Can you work these out from the model? Positions are in its coordinate system, mm. A direction names the side the tool comes from. Round coordinates to 2 decimals unless told otherwise and drop trailing zeros. Loops run counter-clockwise (first coordinate to the right, second up) from the corner with the lowest first, then second, coordinate; pieces in that order, holes last.
(1) If I drill on line 1 along X through (y, z) = (-6.5, -4.25); line 2 along Z through (x, y) = (6.5, -4.5); line 3 along X through (y, z) = (-7.5, -4), over which ranges is the centre line in solid material (lowest first)?
(2) I want a section at D-D on y = -0.5. Write out the boundary of the cut face in (x, z).
(3) Will this pin go through, and if not, where does the flat tip stop? pin 1 Ø1.5 at (x, y) = (-5, -6.5) entering from -Z.
(4) I want a section at A-A on z = -6. Write out the boundary of the cut face in (x, y), plus the area to 3 significant figures.
(5) I want a section at B-B on x = -1. Write out the boundary of the cut face in (y, z), plus the area to 3 significant figures.
(6) I want a section at C-C on y = -3.75. Write out the boundary of the cut face in (x, z).
(7) Thinking about a two-plate mould opening in X: for faces 1 (the face through (-12.458, -7.699, -7.715)), 2 (the face through (0.105, -7.715, 0.301)), 3 (the face through (16.199, -0.285, 0.098)), which applies, released by +X, released by -X, zero draft, split by the parting line, or undercut?
(8) Which directions (+Z, -Z, +X, -X, +Y, -Y) give clear straight access to the entire face, cutting with the end or side of a thin tool? Please do faces 4 (the face through (0, -4, 0)), 5 (the face through (0, 0, 2)), 6 (the face through (8.801, -0.285, -3.958)).
from build123d import *

# Parameters (mm, degrees)
F0_W     = 33
F0_H     = 16
F1_DEPTH = 8
F2_W     = 17
F2_H     = 8
F3_DEPTH = 25
F4_R     = 1


with BuildPart() as f1:
    # F0 (on Front) → F1 (new body)
    with BuildSketch(Plane.XZ):
        Rectangle(F0_W, F0_H)
    extrude(amount=F1_DEPTH)

    # F2 (on face) → F3 (cut)
    with BuildSketch(Plane.XZ.offset(8)):
        with Locations((0, -4)):
            Rectangle(F2_W, F2_H)
    extrude(amount=-F3_DEPTH, mode=Mode.SUBTRACT)

    # F4
    f4_edges = [f1.edges().sort_by_distance(p)[0] for p in [
        (16.5, -8, 0),
        (12.5, -8, -8),
        (8.5, -8, -4),
        (0, -8, 0),
        (-8.5, -8, -4),
        (-12.5, -8, -8),
        (-16.5, -8, 0),
        (0, -8, 8),
        (-8.5, 0, -4),
        (16.5, 0, 0),
        (12.5, 0, -8),
        (8.5, 0, -4),
        (0, 0, 0),
        (-12.5, 0, -8),
        (-16.5, 0, 0),
        (0, 0, 8),
        (-8.5, -4, 0),
        (8.5, -4, 0),
        (-8.5, -4, -8),
        (-16.5, -4, -8),
        (16.5, -4, -8),
        (8.5, -4, -8),
        (16.5, -4, 8),
        (-16.5, -4, 8),
    ]]
    fillet(f4_edges, radius=F4_R)


solid = f1.part
Filled sheet:
1. line 1: x = -16.5 to -8.5, 8.5 to 16.5
1. line 2: z = 0 to 8
1. line 3: x = -16.37 to -8.63, 8.63 to 16.37
2. outline: (-16.37, -7) arc R0.87 ccw to (-15.5, -7.87) - (-9.5, -7.87) arc R0.87 ccw to (-8.63, -7) - (-8.63, -1) arc R1.13 cw to (-7.5, 0.13) - (7.5, 0.13) arc R1.13 cw to (8.63, -1) - (8.63, -7) arc R0.87 ccw to (9.5, -7.87) - (15.5, -7.87) arc R0.87 ccw to (16.37, -7) - (16.37, 7) arc R0.87 ccw to (15.5, 7.87) - (-15.5, 7.87) arc R0.87 ccw to (-16.37, 7) - close
3. pin 1: stops at z = 0
4. outline: (-16.5, -7) arc R1 ccw to (-15.5, -8) - (-9.5, -8) arc R1 ccw to (-8.5, -7) - (-8.5, -1) arc R1 ccw to (-9.5, 0) - (-15.5, 0) arc R1 ccw to (-16.5, -1) - close; (8.5, -7) arc R1 ccw to (9.5, -8) - (15.5, -8) arc R1 ccw to (16.5, -7) - (16.5, -1) arc R1 ccw to (15.5, 0) - (9.5, 0) arc R1 ccw to (8.5, -1) - close
4. area: 126 mm2
5. outline: (-8, 1) arc R1 ccw to (-7, 0) - (-1, 0) arc R1 ccw to (0, 1) - (0, 7) arc R1 ccw to (-1, 8) - (-7, 8) arc R1 ccw to (-8, 7) - close
5. area: 63.1 mm2
6. outline: (-16.5, -7) arc R1 ccw to (-15.5, -8) - (-9.5, -8) arc R1 ccw to (-8.5, -7) - (-8.5, -1) arc R1 cw to (-7.5, 0) - (7.5, 0) arc R1 cw to (8.5, -1) - (8.5, -7) arc R1 ccw to (9.5, -8) - (15.5, -8) arc R1 ccw to (16.5, -7) - (16.5, 7) arc R1 ccw to (15.5, 8) - (-15.5, 8) arc R1 ccw to (-16.5, 7) - close
7. face 1: zero draft
7. face 2: undercut
7. face 3: released by +X
8. face 4: -Z, +Y, -Y
8. face 5: +Z, -Z, +X, -X, +Y
8. face 6: -Z, +Y
